The figure shows three views and two pictorial views of one solid part (mm, origin at its lowest corner). Answer the questions. Round coordinates to 2 decimals unless told otherwise and drop trailing zeros. Order: outer loops, then holes, each group sorted by start corner. A loop starts at its lowest first (then second) coordinate and runs counter-clockwise, first axis right, second up. Notation, with made-up numbers: (-7.75, 64) -> (51.25, 64) arc R15 cw to (51.25, 77) -> close; hole circle Ø2 at (-7, 39.25). An arc over 180 degrees is marked (long way). Return JSON: item names as keys, results as strings. Group by question number.
(1) The part is cut by section B-B (x = 74.5). Determine the outline of the cut face in (y, z), plus the area to 3 significant figures.
(2) Determine the mould class of the marked faces 1, 2 and 3 for opening direction Z: +Z half, -Z half, draft (parallel to the pull), parting line (faces both ways), or undercut.
(3) Consider line 1 (X direction, y = 2.5, z = 24); line 2 (Z direction, x = 30, y = 5); line 3 (Y direction, x = 37, z = 9). Determine where each line is inside the solid, lowest interval first. Write a range as [from, to].
(4) The part is cut by section C-C (z = 9.5). Determine the outline of the cut face in (x, y).
(5) The part is cut by section A-A (y = 1). Determine the outline of the cut face in (x, z), plus the area to 3 significant figures.
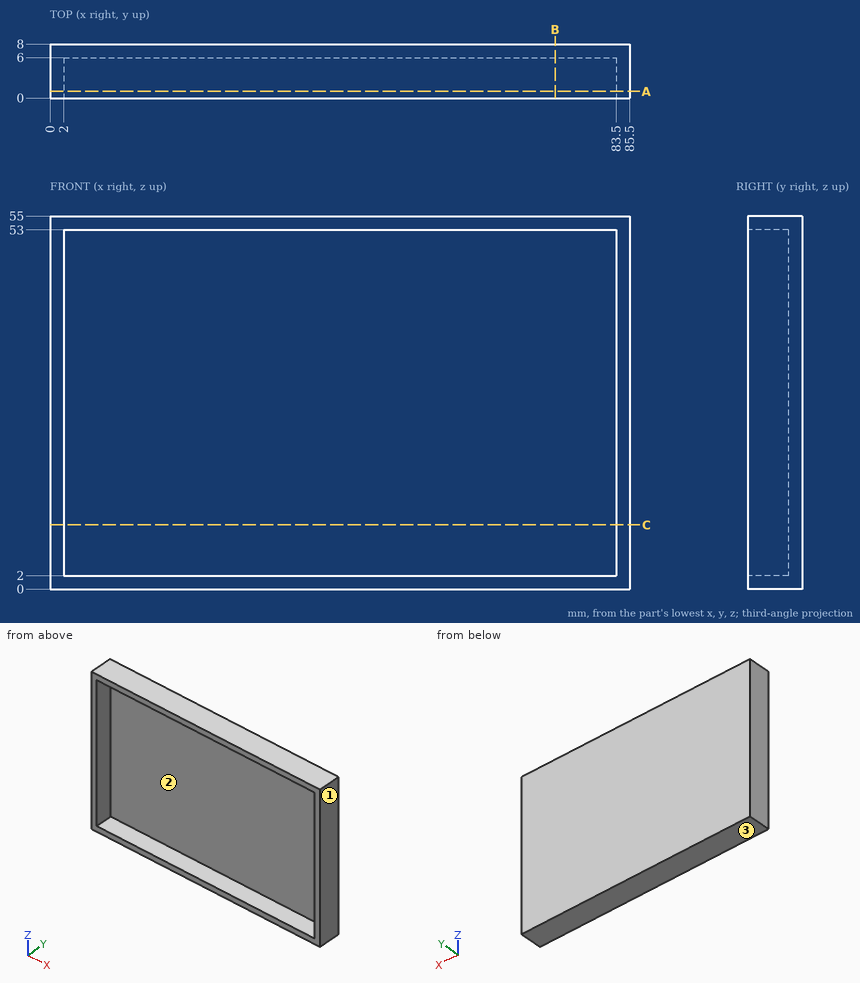
Answer below:
{
 "1": {"outline": "(0, 0) -> (8, 0) -> (8, 55) -> (0, 55) -> (0, 53) -> (6, 53) -> (6, 2) -> (0, 2) -> close", "area": "134 mm²"},
 "2": {"face 1": "draft", "face 2": "undercut", "face 3": "-Z half"},
 "3": {"line 1": "x = [0, 2], [83.5, 85.5]", "line 2": "z = [0, 2], [53, 55]", "line 3": "y = [6, 8]"},
 "4": {"outline": "(0, 0) -> (2, 0) -> (2, 6) -> (83.5, 6) -> (83.5, 0) -> (85.5, 0) -> (85.5, 8) -> (0, 8) -> close"},
 "5": {"outline": "(0, 0) -> (85.5, 0) -> (85.5, 55) -> (0, 55) -> close; hole (2, 2) -> (83.5, 2) -> (83.5, 53) -> (2, 53) -> close", "area": "546 mm²"}
}
